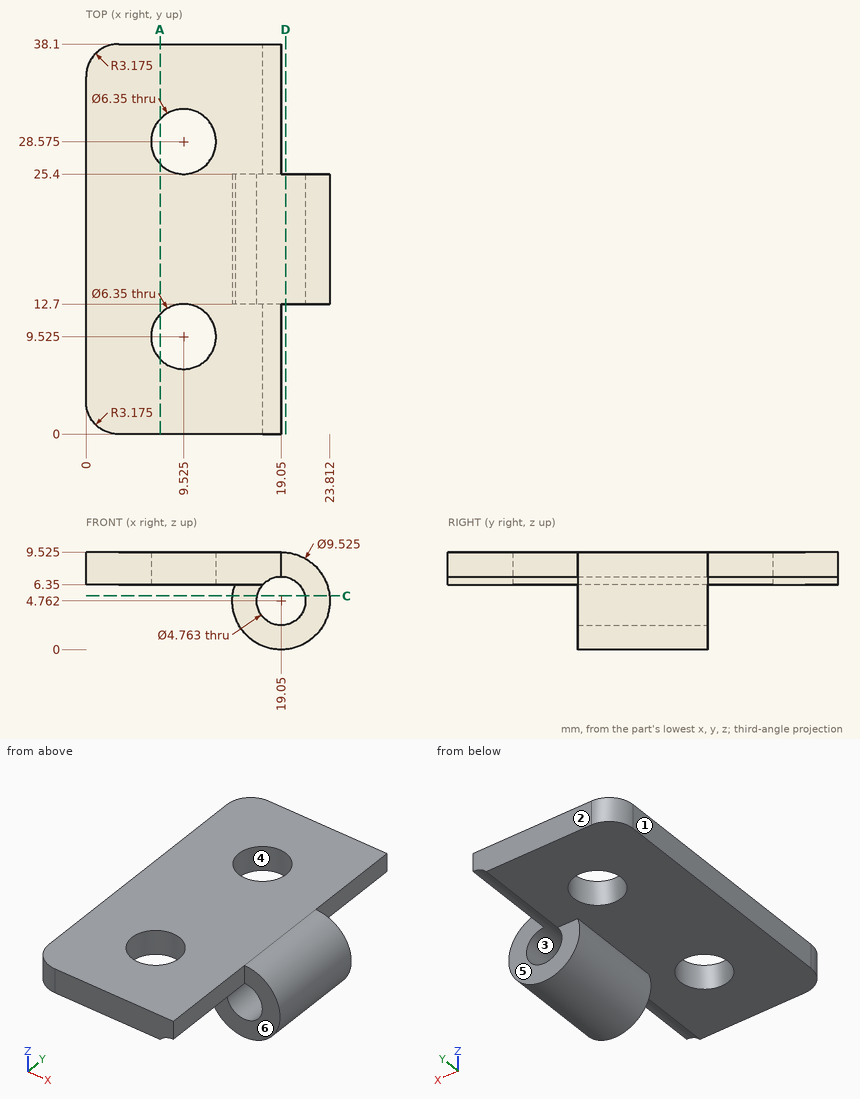
Part print with two shaded views. Sizes in mm from the minimum x, y, z corner. A direction names the side the tool comes from. Give positions to 0.01 mm unless a question says otherwise; leave off trailing zeros. Order: outer loops, then holes, each group sorted by start corner. A loop starts at its lowest first (then second) coordinate and runs counter-clockwise, first axis right, second up. Notation, with made-up numbers: (64, 68.5) - (93, 68.5) arc R36 ccw to (93, 102.5) - close; hole circle Ø7 at (14, 54.5). An arc over 180 degrees is marked (long way). Write each question's results on one line, items separated by ' | '.
1. Pull direction X, two halves, no side cores. Call the marked faces 1, 2 and 3: released by +X, released by -X, zero draft, split by the parting line, or undercut.
Calculated:
face 1: released by -X | face 2: zero draft | face 3: undercut
2. Saw through at A-A on x = 7.25. Count the separate pieces of the cut face and the enclosed holes in it.
Calculated:
separate pieces: 3 | enclosed holes: 0
3. Probe L1, parallel to Y at x = 9.75, z = 7.75; L2, parallel to Z at x = 19.05, y = 22.5 (1 decimal); L3, parallel to Y at x = 22.5, z = 2. List the from-to ranges inside material, lowest first. Write a range as from..to.
Calculated:
L1: y = 0..6.36, 12.69..25.41, 31.74..38.1 | L2: z = 0..2.4, 7.1..9.5 | L3: y = 12.7..25.4
4. Saw through at C-C on z = 5.25. List the corners of the cut face in (x, y).
Calculated:
outline: (14.31, 12.7) - (16.72, 12.7) - (16.72, 25.4) - (14.31, 25.4) - close; (21.38, 12.7) - (23.79, 12.7) - (23.79, 25.4) - (21.38, 25.4) - close
5. Pin check, flat tips, straight feed: pin 1 (1.9 mm diameter, centred on y = 31, z = 8.5, fed in from +X); pin 2 (3 mm diameter, centred on x = 18, z = 2.5, fed in from +Y); pin 3 (10 mm diameter, centred on x = 6, y = 19, fed in from -Z); pin 4 (5 mm diameter, centred on x = 3.5, z = 5, fed in from +Y). Stop position of each tip, or through.
Calculated:
pin 1: stops at x = 19.05 | pin 2: stops at y = 25.4 | pin 3: stops at z = 6.35 | pin 4: stops at y = 38.1
6. 3-axis set-ups, long thin cutter, end or side, ignore diameter. For the marked faces 4, 5 and 6: which of +Z, -Z, +X, -X, +Y, -Y reach the whole face in a straight line?
Calculated:
face 4: +Z, -Z | face 5: -Z, +X, +Y | face 6: -Z, +X, -Y
7. Saw through at D-D on x = 19.5. List the corners of the cut face in (y, z) (1 decimal).
Calculated:
outline: (12.7, 0) - (25.4, 0) - (25.4, 2.4) - (12.7, 2.4) - close; (12.7, 7.1) - (25.4, 7.1) - (25.4, 9.5) - (12.7, 9.5) - close
